Read the model definition and answer for the solid it produces. Units are mm, in the model's axes. A direction names the side the tool comes from. Round coordinates to 2 decimals unless told otherwise and drop trailing zeros. Write each loop counter-clockwise with the first axis right and the second up, starting at its lowest first coordinate (ties: lowest second). Pieces come first, ordered by that corner, then holes. Notation, with made-up numbers: (32.25, 9.25) - (67.25, 9.25) arc R37 cw to (67.25, 48.25) - close; hole circle Ø7 at (36, 20). An arc over 180 degrees is marked (long way). Answer as CSV lines item,"result". Start each with the question number.
1) Find section C-C on x = 4. Determine the outline of the cut face in (y, z), then the cut area to 3 significant figures.
2) Find section A-A on y = 0. Determine the outline of the cut face in (x, z), then the cut area to 3 significant figures.
3) Each of these flat-tipped pins is pushed along its axis until it touches: pin 1 (1.1 mm diameter, centred on x = 0.5, z = 0.5, fed in from -Y); pin 2 (1.1 mm diameter, centred on x = 0.5, z = -0.5, fed in from +Y); pin 3 (4 mm diameter, centred on x = 10, z = 2.5, fed in from +Y). Where does it stop, or does it pass through?
4) Consider line 1 along X through (y, z) = (-2.25, -0.5); line 2 along X through (y, z) = (-0.5, 3.75); line 3 along Z through (x, y) = (9.25, -1.5). Determine where each line is inside the solid, lowest interval first.
5) Find section D-D on x = 1.75. Determine the outline of the cut face in (y, z), then the cut area to 3 significant figures.
6) For a pull along Y with two mould halves and no side action, classify faces 4 (the conical face through (1.449, 3.475, 1.807)), 5 (the flat face through (0.5, 0.6, 0.1)), 6 (the flat face through (0.5, -0.6, 0.1)), 7 (the flat face through (12.4, 0, 0)) as +Y half, -Y half, draft (parallel to the pull), parting line (faces both ways), or undercut.
7) Find section B-B on z = 0. Determine the outline of the cut face in (x, y), then the cut area to 3 significant figures.
8) Which of the six approach directions +Z, -Z, +X, -X, +Y, -Y give full straight-line access (tool end or side, diameter ignored) to faces 1 (the flat face through (2.4, -2, -1)), 2 (the flat face through (0, -1, 0)), 3 (the flat face through (1, 0, 0))?
from build123d import *

# Parameters (mm, degrees)
FILLET2_R  = 1.2
SKETCH2_W  = 8
SKETCH2_H  = 1.2
SLOT_DEPTH = 1


with BuildPart() as part:
    # BodySke → Base-Revolve (revolve)
    with BuildSketch(Plane.XY, mode=Mode.PRIVATE) as base_revolve_sk:
        Polygon((2.4, 2), (2.4, 4), (0, 3.790027208), (0, 0), (12.4, 0), (12.4, 2), align=None)
    revolve(base_revolve_sk.sketch.rotate(Axis((-25.4, 0, 0), (1, 0, 0)), 90), axis=Axis((-25.4, 0, 0), (1, 0, 0)))  # turned: the seam where the file's is

    # Fillet2
    fillet2_edges = [part.edges().sort_by_distance(p)[0] for p in [
        (0, 0, -3.790027208),
    ]]
    fillet(fillet2_edges, radius=FILLET2_R)

    # Sketch2 → Slot (cut)
    with BuildSketch(Plane(origin=(0, 0, 0), x_dir=(0, 0, -1), z_dir=(1, 0, 0))):
        Rectangle(SKETCH2_W, SKETCH2_H)
    extrude(amount=SLOT_DEPTH, mode=Mode.SUBTRACT)


solid = part.part
Check values:
1,outline,"circle Ø4 at (0, 0)"
1,area,"12.6 mm^2"
2,outline,"(1, -3.87) arc R1.2 ccw to (1.1, -3.89) - (2.4, -4) - (2.4, -2) - (12.4, -2) - (12.4, 2) - (2.4, 2) - (2.4, 4) - (1.1, 3.89) arc R1.2 ccw to (1, 3.87) - close"
2,area,"51.0 mm^2"
3,pin 1,"stops at y = -3.86"
3,pin 2,"stops at y = 3.86"
3,pin 3,"stops at y = 1.94"
4,line 1,"x = 0 to 2.4"
4,line 2,"x = 1 to 2.4"
4,line 3,"z = -1.32 to 1.32"
5,outline,"circle Ø7.89 at (0, 0)"
5,area,"48.8 mm^2"
6,face 4,"parting line"
6,face 5,"undercut"
6,face 6,"undercut"
6,face 7,"draft"
7,outline,"(0, -2.69) arc R1.2 ccw to (1.1, -3.89) - (2.4, -4) - (2.4, -2) - (12.4, -2) - (12.4, 2) - (2.4, 2) - (2.4, 4) - (1.1, 3.89) arc R1.2 ccw to (0, 2.69) - (0, 0.6) - (1, 0.6) - (1, -0.6) - (0, -0.6) - close"
7,area,"57.0 mm^2"
8,face 1,"+X"
8,face 2,"+Z, -Z, -X, +Y, -Y"
8,face 3,"+Z, -Z, -X"
